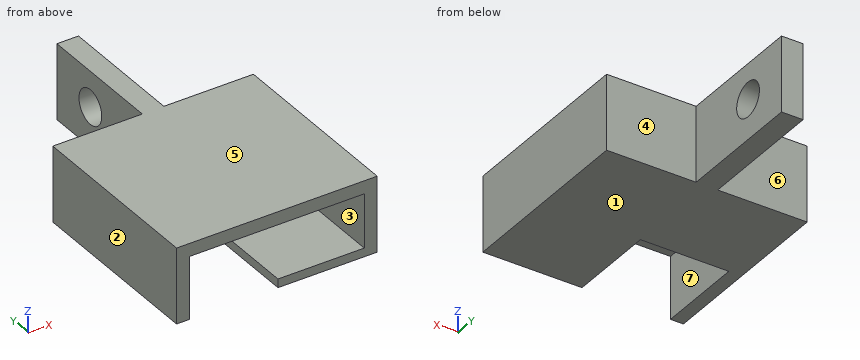
```python
from build123d import *

# Parameters (mm, degrees)
SKETCH_W        = 46.5
SKETCH_H        = 43.5
PAD_DEPTH       = 17.5
SKETCH001_W     = 40.5
SKETCH001_H     = 12.5
POCKET_DEPTH    = 40.5
SKETCH002_W     = 20.5
SKETCH002_H     = 20.5
POCKET001_DEPTH = 3
SKETCH003_W     = 5
SKETCH003_H     = 30
PAD001_DEPTH    = 17.5
SKETCH004_R     = 4
POCKET002_DEPTH = 5
POCKET003_DEPTH = 100


with BuildPart() as part:
    # Sketch → Pad (new body)
    with BuildSketch(Plane.XY):
        Rectangle(SKETCH_W, SKETCH_H)
    extrude(amount=PAD_DEPTH)

    # Sketch001 (on Face3 of Pad) → Pocket (cut)
    with BuildSketch(Plane.XZ.offset(21.75)):
        with Locations((0, 8.25)):
            Rectangle(SKETCH001_W, SKETCH001_H)
    extrude(amount=-POCKET_DEPTH, mode=Mode.SUBTRACT)

    # Sketch002 (on Face4 of Pocket) → Pocket001 (cut)
    with BuildSketch(Plane(origin=(0, 0, 0), x_dir=(1, 0, 0), z_dir=(0, 0, -1))):
        with Locations((-10, 11.5)):
            Rectangle(SKETCH002_W, SKETCH002_H)
    extrude(amount=-POCKET001_DEPTH, mode=Mode.SUBTRACT)

    # Sketch003 (on Face5 of Pocket001) → Pad001 (join)
    with BuildSketch(Plane.XY.offset(17.5)):
        with Locations((0, 36.75)):
            Rectangle(SKETCH003_W, SKETCH003_H)
    extrude(amount=-PAD001_DEPTH)

    # Sketch004 (on Face19 of Pad001) → Pocket002 (cut)
    with BuildSketch(Plane.YZ.offset(-20.25)):
        with Locations((40, 9.25)):
            Circle(SKETCH004_R)
    extrude(amount=-POCKET002_DEPTH, mode=Mode.SUBTRACT)

    # Sketch004 (on Face19 of Pad001) → Pocket003 (cut)
    with BuildSketch(Plane.YZ.offset(-20.25)):
        with Locations((40, 9.25)):
            Circle(SKETCH004_R)
    extrude(amount=POCKET003_DEPTH, mode=Mode.SUBTRACT)


solid = part.part
```
Input: part model. Units: mm. Frame: model coordinates. Face numbers are marked on the shaded views. A direction names the side the tool comes from. Coordinates: 2 decimals unless noted, no trailing zeros. Write each loop counter-clockwise with the first axis right and the second up, starting at its lowest first coordinate (ties: lowest second). Pieces come first, ordered by that corner, then holes. Notation, with made-up numbers: (3.25, 40) -> (24.25, 40) arc R29 cw to (24.25, 60) -> close; hole circle Ø3 at (78, 22.5). An arc over 180 degrees is marked (long way). Answer as a JSON object with one key per item and string values.
1. Mould query, pull axis Z, two halves, no side actions, for the marked faces 1, 2 and 3. Classes: released by +Z, released by -Z, zero draft, split by the parting line, or undercut.
Result set:
{"face 1": "released by -Z", "face 2": "zero draft", "face 3": "undercut"}
2. Section C-C on x = -0.5. Return the cut outline in (y, z), then the cut area to 3 significant figures.
Result set:
{"outline": "(-21.75, 14.5) -> (18.75, 14.5) -> (18.75, 2) -> (-1.25, 2) -> (-1.25, 0) -> (51.75, 0) -> (51.75, 17.5) -> (-21.75, 17.5) -> close; hole circle Ø8 at (40, 9.25)", "area": "689 mm2"}
3. First-contact query: P1, Ø5, axis at x = -12, y = 26.5, coming from the -Z side; P2, Ø5, axis at y = 33.5, z = 6.5, coming from the -X side; P3, Ø2, axis at x = -11.5, z = 6.5, coming from the +Y side; P4, Ø1.6, axis at x = -5.5, z = 0.5, coming from the -Y side. Flat tips, straight axial feed; report the tip coordinate or a pass-through.
Result set:
{"P1": "passes through", "P2": "stops at x = -2.5", "P3": "stops at y = 21.75", "P4": "stops at y = -1.25"}
4. Material intervals for line 1 (Z direction, x = -0.8, y = 40); line 2 (X direction, y = -2, z = 2.75); line 3 (Y direction, x = 0.35, z = 9.25), sorted ascending. Write a range as from..to.
Result set:
{"line 1": "z = 0..5.25, 13.25..17.5", "line 2": "x = -23.25..-20.25, 20.25..23.25", "line 3": "y = 18.75..36, 44..51.75"}
5. Section D-D on z = 4.25. Return the cut outline in (x, y).
Result set:
{"outline": "(-23.25, -21.75) -> (-20.25, -21.75) -> (-20.25, 18.75) -> (20.25, 18.75) -> (20.25, -21.75) -> (23.25, -21.75) -> (23.25, 21.75) -> (2.5, 21.75) -> (2.5, 51.75) -> (-2.5, 51.75) -> (-2.5, 21.75) -> (-23.25, 21.75) -> close"}
6. Section B-B on y = 8. Return the cut outline in (x, z), then the cut area to 4 significant figures.
Result set:
{"outline": "(-23.25, 0) -> (23.25, 0) -> (23.25, 17.5) -> (-23.25, 17.5) -> close; hole (-20.25, 2) -> (20.25, 2) -> (20.25, 14.5) -> (-20.25, 14.5) -> close", "area": "307.5 mm2"}
7. Access query for the marked faces 4, 5, 6 and 7. Directions: +Z, -Z, +X, -X, +Y, -Y. A direction counts if a zero-diameter tool reaches every point of the face in a straight line with its end or side. Return the directions, or none.
Result set:
{"face 4": "+Z, -Z, +X, +Y", "face 5": "+Z, +X, -X, +Y, -Y", "face 6": "+Z, -Z, -X, +Y", "face 7": "-Y"}
8. Section A-A on z = 9.25. Return the cut outline in (x, y), then the cut area to 4 significant figures.
Result set:
{"outline": "(-23.25, -21.75) -> (-20.25, -21.75) -> (-20.25, 18.75) -> (20.25, 18.75) -> (20.25, -21.75) -> (23.25, -21.75) -> (23.25, 21.75) -> (2.5, 21.75) -> (2.5, 36) -> (-2.5, 36) -> (-2.5, 21.75) -> (-23.25, 21.75) -> close; (-2.5, 44) -> (2.5, 44) -> (2.5, 51.75) -> (-2.5, 51.75) -> close", "area": "492.5 mm2"}
